Input: part model. Units: mm. Frame: model coordinates. Face numbers are marked on the shaded views. A direction names the side the tool comes from. Round coordinates to 2 decimals unless told otherwise and drop trailing zeros. Loops run counter-clockwise (first coordinate to the right, second up) from the corner with the lowest first, then second, coordinate; pieces in that order, holes last. Notation, with made-up numbers: (-9, 7.5) - (22, 7.5) arc R34 cw to (22, 46.5) - close; hole circle Ø10 at (61, -22.75). An arc over 180 degrees is marked (long way). One line per question, with ' | ' between items. Start each with the question number.
from build123d import *

# Parameters (mm, degrees)
F1_DEPTH = 50.8
F0_W     = 68.1800022721
F0_H     = 33.179204911
F2_DEPTH = 12.7


with BuildPart() as f1:
    # F0 (on Front) → F1 (new body)
    with BuildSketch(Plane.XZ):
        Polygon((-77.840000391, 0), (-68.1800022721, 0), (-68.1800022721, 33.179204911), (0, 33.179204911), (0, 39.4792035222), (-77.840000391, 39.4792035222), align=None)
        Polygon((-68.1800022721, -33.179204911), (-68.1800022721, 0), (-77.840000391, 0), (-77.840000391, -39.4792035222), (0, -39.4792035222), (0, -33.179204911), align=None)
        Polygon((0, 39.4792035222), (0, 33.179204911), (68.1800022721, 33.179204911), (68.1800022721, 0), (77.840000391, 0), (77.840000391, 39.4792035222), align=None)
        Polygon((77.840000391, 0), (68.1800022721, 0), (68.1800022721, -33.179204911), (0, -33.179204911), (0, -39.4792035222), (77.840000391, -39.4792035222), align=None)
    extrude(amount=F1_DEPTH)

    # F0 (on Front) → F2 (join)
    with BuildSketch(Plane.XZ):
        with Locations((-34.0900011361, 16.5896024555)):
            Rectangle(F0_W, F0_H)
        with Locations((34.0900011361, 16.5896024555)):
            Rectangle(F0_W, F0_H)
        with Locations((34.0900011361, -16.5896024555)):
            Rectangle(F0_W, F0_H)
        with Locations((-34.0900011361, -16.5896024555)):
            Rectangle(F0_W, F0_H)
    extrude(amount=F2_DEPTH)


solid = f1.part
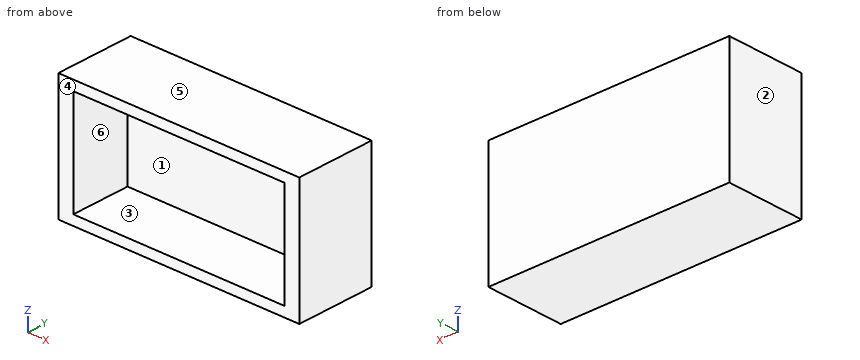
(1) Section B-B, the plane x = 25.5. Output: boundary loops of the cut face in (y, z), plus the area to 3 significant figures.
(2) Pin query (flat end, axial travel): P1, Ø5, axis at x = 27, z = -21.5, coming from the +Y side; P2, Ø3, axis at x = 35.5, z = 27.5, coming from the -Y side. Return the tip coordinate at first contact, or that it passes through.
(3) Line query: line 1 along Z through (x, y) = (43, -30); line 2 along X through (y, z) = (-20, 19); line 3 along Y through (x, z) = (-64, -29). Output: solid intervals per line, ascending. Write a range as from..to.
(4) Section C-C, the plane z = -31.5. Output: boundary loops of the cut face in (x, y).
(5) Pull-direction query (X, two-part tool) for the marked faces 1, 2, 3 and 4; classes: released by +X, released by -X, zero draft, split by the parting line, or undercut.
(6) Section A-A, the plane y = -17.5. Output: boundary loops of the cut face in (x, z), plus the area to 3 significant figures.
(7) Reachability of the marked faces 5 and 6 from +Z, -Z, +X, -X, +Y, -Y: full face, straight path, thin tool, end or side. Return the list, or none.
Derived:
1) outline: (-50.8, -39.48) - (0, -39.48) - (0, 39.48) - (-50.8, 39.48) - (-50.8, 33.18) - (-12.7, 33.18) - (-12.7, -33.18) - (-50.8, -33.18) - close | area: 1,480 mm²
2) P1: stops at y = 0 | P2: stops at y = -12.7
3) line 1: z = -39.48..-33.18, 33.18..39.48 | line 2: x = -77.84..-68.18, 68.18..77.84 | line 3: y = -12.7..0
4) outline: (-77.84, -50.8) - (-68.18, -50.8) - (-68.18, -12.7) - (68.18, -12.7) - (68.18, -50.8) - (77.84, -50.8) - (77.84, 0) - (-77.84, 0) - close
5) face 1: undercut | face 2: released by -X | face 3: undercut | face 4: zero draft
6) outline: (-77.84, -39.48) - (77.84, -39.48) - (77.84, 39.48) - (-77.84, 39.48) - close; hole (-68.18, -33.18) - (68.18, -33.18) - (68.18, 33.18) - (-68.18, 33.18) - close | area: 3,240 mm²
7) face 5: +Z, +X, -X, +Y, -Y | face 6: -Y
